The model under review builds one solid part; all positions refer to its coordinate system, in mm. A direction names the side the tool comes from. Give positions to 0.01 mm unless a question says otherwise; leave off trailing zeros. Order: outer loops, then holes, each group sorted by start corner. A loop starts at its lowest first (then second) coordinate and runs counter-clockwise, first axis right, second up. Notation, with made-up numbers: (85, -5.5) - (126, -5.5) arc R28 ccw to (126, 22.5) - close; hole circle Ø11 at (43, -35). An arc over 180 degrees is marked (long way). Put each result on its own line as item: value.
```python
from build123d import *

# Parameters (mm, degrees)
DODANIE_WYCI_GNI_CIE1_DEPTH = 1810
SZKIC2_W                    = 172.684782789
SZKIC2_H                    = 104.540186521
WYTNIJ_WYCI_GNI_CIE1_DEPTH  = 1324.650255921
SZKIC3_W                    = 177.628833627
SZKIC3_H                    = 120.563010223
WYTNIJ_WYCI_GNI_CIE2_DEPTH  = 1782.263596439


with BuildPart() as part:
    # Szkic1 → Dodanie-wyciągnięcie1 (new body)
    with BuildSketch(Plane(origin=(0, 0, 0), x_dir=(1, 0, 0), z_dir=(0, 1, 0))):
        with BuildLine():
            ThreePointArc((0, 57), (0.878679656, 59.121320344), (3, 60))
            Line((3, 60), (57, 60))
            ThreePointArc((57, 60), (59.121320344, 59.121320344), (60, 57))
            Line((60, 57), (60, 3))
            ThreePointArc((60, 3), (59.121320344, 0.878679656), (57, 0))
            Line((57, 0), (3, 0))
            ThreePointArc((3, 0), (0.878679656, 0.878679656), (0, 3))
            Line((0, 3), (0, 57))
        make_face()
        with BuildLine():
            Line((3, 6), (3, 54))
            ThreePointArc((3, 54), (3.878679656, 56.121320344), (6, 57))
            Line((6, 57), (54, 57))
            ThreePointArc((54, 57), (56.121320344, 56.121320344), (57, 54))
            Line((57, 54), (57, 6))
            ThreePointArc((57, 6), (56.121320344, 3.878679656), (54, 3))
            Line((54, 3), (6, 3))
            ThreePointArc((6, 3), (3.878679656, 3.878679656), (3, 6))
        make_face(mode=Mode.SUBTRACT)
    extrude(amount=DODANIE_WYCI_GNI_CIE1_DEPTH)

    # Szkic2 → Wytnij-wyciągnięcie1 (cut, through all)
    with BuildSketch(Plane(origin=(0, 875, 875), x_dir=(1, 0, 0), z_dir=(0, 0.7071067811865464, 0.7071067811865488))):
        with Locations((31.260805739, 1283.757898566)):
            Rectangle(SZKIC2_W, SZKIC2_H)
    extrude(amount=WYTNIJ_WYCI_GNI_CIE1_DEPTH, mode=Mode.SUBTRACT)

    # Szkic3 → Wytnij-wyciągnięcie2 (cut, through all)
    with BuildSketch(Plane(origin=(0, 30, -30), x_dir=(1, 0, 0), z_dir=(0, -0.7071067811865464, 0.7071067811865488))):
        with Locations((21.62509475, 2.040675712)):
            Rectangle(SZKIC3_W, SZKIC3_H)
    extrude(amount=WYTNIJ_WYCI_GNI_CIE2_DEPTH, mode=Mode.SUBTRACT)


solid = part.part
```
(1) Take a section at A-A, the plane z = -43.5. Write out the cut boundary in (x, y), then the cut area to 3 significant figures.
The answers:
outline: (0, 16.5) - (3, 16.5) - (3, 1793.5) - (0, 1793.5) - close; (57, 16.5) - (60, 16.5) - (60, 1793.5) - (57, 1793.5) - close
area: 10,700 mm^2
(2) The part is to be moulded in two halves that separate along X. For faces 1 (the flat face through (60, 892, -30)), 2 (the flat face through (3, 892, -30)), 3 (the flat face through (30, 892, -60)), say which applies: pulls with the +X half, pulls with the -X half, needs draft (parallel to the pull), parting line crosses it, or undercut.
The answers:
face 1: pulls with the +X half
face 2: undercut
face 3: needs draft
(3) For faces 4 (the flat face through (30, 892, -57)), 5 (the flat face through (1, 32, -28)), list the 3-axis set-ups (+Z, -Z, +X, -X, +Y, -Y) from which the entire face can be reached by the end or side of a thin tool; tool diameter is ignored.
The answers:
face 4: +Y, -Y
face 5: +Z, +X, -X, -Y
(4) Take a section at C-C, the plane x = 29.5. Write out the cut boundary in (y, z).
The answers:
outline: (0, -60) - (1810, -60) - (1807, -57) - (3, -57) - close; (57, -3) - (1753, -3) - (1750, 0) - (60, 0) - close
(5) Wall thickness on L1, parallel to Z at x = 26, y = 1253.5; L2, parallel to X at y = 1167.5, z = -30; L3, parallel to X at y = 228.5, z = -55: over which ranges is each line inside the solid? List them lowest first.
The answers:
L1: -60 to -57, -3 to 0
L2: 0 to 3, 57 to 60
L3: 0 to 3.17, 56.83 to 60
(6) Clearance check with a flat-ended pin moving along its axis: pin 1 Ø10 at (x, z) = (47.5, -21.5) entering from -Y. State where the tip first meets the part, or that it passes through.
The answers:
pin 1: through
(7) Take a section at B-B, the plane y = 337.5. Write out the cut boundary in (x, z).
The answers:
outline: (0, -57) arc R3 ccw to (3, -60) - (57, -60) arc R3 ccw to (60, -57) - (60, -3) arc R3 ccw to (57, 0) - (3, 0) arc R3 ccw to (0, -3) - close; hole (3, -54) arc R3 ccw to (6, -57) - (54, -57) arc R3 ccw to (57, -54) - (57, -6) arc R3 ccw to (54, -3) - (6, -3) arc R3 ccw to (3, -6) - close
